Input: part model. Units: mm. Frame: model coordinates. Coordinates: 2 decimals unless noted, no trailing zeros. Loops run counter-clockwise (first coordinate to the right, second up) from the corner with the lowest first, then second, coordinate; pieces in that order, holes last.
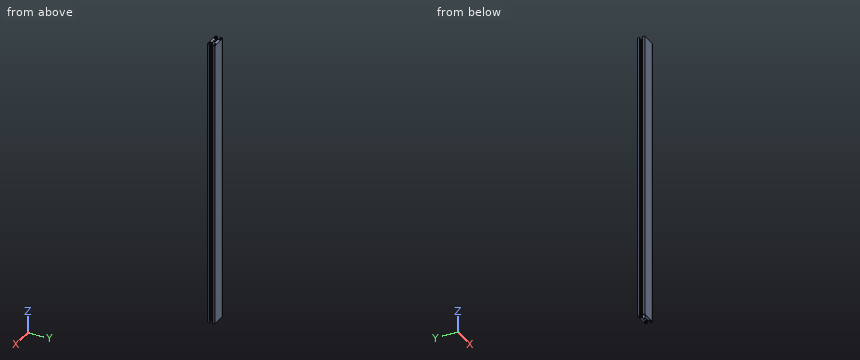
```python
from build123d import *

# Parameters (mm, degrees)
SKETCH1_R           = 3.25
BOSS_EXTRUDE1_DEPTH = 400


with BuildPart() as part:
    # Sketch1 → Boss-Extrude1 (new, symmetric)
    with BuildSketch(Plane.XY):
        with BuildLine():
            Line((1.5, 0), (38.5, 0))
            ThreePointArc((38.5, 0), (39.560660172, 0.439339828), (40, 1.5))
            Line((40, 1.5), (40, 5.5))
            ThreePointArc((40, 5.5), (39.853553391, 5.853553391), (39.5, 6))
            Line((39.5, 6), (37.5, 6))
            ThreePointArc((37.5, 6), (37.146446609, 5.853553391), (37, 5.5))
            Line((37, 5.5), (37, 2.5))
            ThreePointArc((37, 2.5), (36.853553391, 2.146446609), (36.5, 2))
            Line((36.5, 2), (29.5, 2))
            ThreePointArc((29.5, 2), (29.146446609, 2.146446609), (29, 2.5))
            Line((29, 2.5), (29, 5.5))
            ThreePointArc((29, 5.5), (28.853553391, 5.853553391), (28.5, 6))
            Line((28.5, 6), (26.5, 6))
            ThreePointArc((26.5, 6), (26.146446609, 6.146446609), (26, 6.5))
            Line((26, 6.5), (26, 13.5))
            ThreePointArc((26, 13.5), (26.146446609, 13.853553391), (26.5, 14))
            Line((26.5, 14), (28.5, 14))
            ThreePointArc((28.5, 14), (28.853553391, 14.146446609), (29, 14.5))
            Line((29, 14.5), (29, 17.5))
            ThreePointArc((29, 17.5), (29.146446609, 17.853553391), (29.5, 18))
            Line((29.5, 18), (36.5, 18))
            ThreePointArc((36.5, 18), (36.853553391, 17.853553391), (37, 17.5))
            Line((37, 17.5), (37, 14.5))
            ThreePointArc((37, 14.5), (37.146446609, 14.146446609), (37.5, 14))
            Line((37.5, 14), (39.5, 14))
            ThreePointArc((39.5, 14), (39.853553391, 14.146446609), (40, 14.5))
            Line((40, 14.5), (40, 18.5))
            ThreePointArc((40, 18.5), (39.560660172, 19.560660172), (38.5, 20))
            Line((38.5, 20), (1.5, 20))
            ThreePointArc((1.5, 20), (0.439339828, 19.560660172), (0, 18.5))
            Line((0, 18.5), (0, 14.5))
            ThreePointArc((0, 14.5), (0.146446609, 14.146446609), (0.5, 14))
            Line((0.5, 14), (2.5, 14))
            ThreePointArc((2.5, 14), (2.853553391, 14.146446609), (3, 14.5))
            Line((3, 14.5), (3, 17.5))
            ThreePointArc((3, 17.5), (3.146446609, 17.853553391), (3.5, 18))
            Line((3.5, 18), (10.5, 18))
            ThreePointArc((10.5, 18), (10.853553391, 17.853553391), (11, 17.5))
            Line((11, 17.5), (11, 14.5))
            ThreePointArc((11, 14.5), (11.146446609, 14.146446609), (11.5, 14))
            Line((11.5, 14), (13.5, 14))
            ThreePointArc((13.5, 14), (13.853553391, 13.853553391), (14, 13.5))
            Line((14, 13.5), (14, 6.5))
            ThreePointArc((14, 6.5), (13.853553391, 6.146446609), (13.5, 6))
            Line((13.5, 6), (11.5, 6))
            ThreePointArc((11.5, 6), (11.146446609, 5.853553391), (11, 5.5))
            Line((11, 5.5), (11, 2.5))
            ThreePointArc((11, 2.5), (10.853553391, 2.146446609), (10.5, 2))
            Line((10.5, 2), (3.5, 2))
            ThreePointArc((3.5, 2), (3.146446609, 2.146446609), (3, 2.5))
            Line((3, 2.5), (3, 5.5))
            ThreePointArc((3, 5.5), (2.853553391, 5.853553391), (2.5, 6))
            Line((2.5, 6), (0.5, 6))
            ThreePointArc((0.5, 6), (0.146446609, 5.853553391), (0, 5.5))
            Line((0, 5.5), (0, 1.5))
            ThreePointArc((0, 1.5), (0.439339828, 0.439339828), (1.5, 0))
        make_face()
        with Locations((20, 10)):
            Circle(SKETCH1_R, mode=Mode.SUBTRACT)
    extrude(amount=BOSS_EXTRUDE1_DEPTH, both=True)


solid = part.part
```
Item 1: Line query: L1, parallel to X at y = 4, z = 55; L2, parallel to Y at x = 20, z = 154.5; L3, parallel to X at y = 10.25, z = 85. Output: solid intervals per line, ascending.
Result:
L1: x = 0 to 3, 11 to 29, 37 to 40
L2: y = 0 to 6.75, 13.25 to 20
L3: x = 14 to 16.76, 23.24 to 26
Item 2: Contact query for flat-ended pins moving along their axis: P1, Ø3, axis at y = 10, z = 146, coming from the -X side; P2, Ø3.5, axis at y = 9.5, z = -33.5, coming from the +X side. Output: stop coordinate, or through.
Result:
P1: stops at x = 14
P2: stops at x = 26
Item 3: Section query A-A (y = 10). Output: boundary loops of the cut face in (x, z), then the cut area to 3 significant figures.
Result:
outline: (14, -400) - (16.75, -400) - (16.75, 400) - (14, 400) - close; (23.25, -400) - (26, -400) - (26, 400) - (23.25, 400) - close
area: 4,400 mm2
